Autodesk Inventor part; units mm, degrees
ref_plane "YZ Plane" through (0, 0, 0) normal (1, 0, 0) x (0, 1, 0)
ref_plane "XZ Plane" through (0, 0, 0) normal (0, 1, 0) x (-1, 0, 0)
ref_plane "XY Plane" through (0, 0, 0) normal (0, 0, 1) x (1, 0, 0)
ref_plane "Work Plane1" through (0, 0, 0) normal (0, 0, 1) x (1, 0, 0)
sketch "Sketch1" plane through (0, 0, 0) normal (0, 0, 1) x (1, 0, 0)
  circle A0 centre (0, -11.4) radius 0.5 construction
  circle A1 centre (0, 8.1) radius 0.5 construction
  circle A2 centre (0, -1.6) radius 3.9462 construction
  line L0 (8.2, 14.1) -> (-8.2, 14.1) construction
  line L1 (-8.2, 14.1) -> (-8.2, -14.1) construction
  line L2 (-8.2, -14.1) -> (8.2, -14.1) construction
  line L3 (8.2, -14.1) -> (8.2, 14.1) construction
  line L4 (-4, -9.1) -> (4, -9.1)
  line L5 (4, -9.1) -> (4, 5.9)
  line L6 (4, 5.9) -> (-4, 5.9)
  line L7 (-4, 5.9) -> (-4, -9.1)
  line L8 (-4, -9.1) -> (4, 5.9) construction
  line L9 (4, -9.1) -> (-4, 5.9) construction
  circle A3 centre (13, 11.4) radius 1.45 construction
  circle A4 centre (13, -14.6) radius 1.45 construction
  circle A5 centre (-20, -1.6) radius 1.45 construction
  line L10 (16, -17.6) -> (16, 14.4) construction
  line L11 (16, 14.4) -> (-16, 14.4) construction
  line L12 (-16, -17.6) -> (16, -17.6) construction
  line L13 (16, 14.4) -> (-24, 14.4)
  line L14 (-24, 14.4) -> (-24, -17.6)
  line L15 (-24, -17.6) -> (16, -17.6)
  line L16 (16, -17.6) -> (16, 14.4)
  circle A6 centre (0, 8.1) radius 0.5
  circle A7 centre (0, -11.4) radius 0.5
  point P0 (0, 0)
extrude "Extrusion1" add sketch "Sketch1" along normal blind 5
ref_plane "Work Plane2" through (-24, -1.6, 0) normal (0, -1, 0) x (1, 0, 0)
sketch "Sketch2" plane through (-24, -1.6, 0) normal (0, -1, 0) x (1, 0, 0)
  line L0 (1, 9) -> (1, 5)
  line L1 (7, 9) -> (7, 5)
  circle A0 centre (4, 4) radius 2.55
  line L2 (4, 6.55) -> (4, 1.45)
  point P0 (24, 0)
  dimension "d6" = 5.1
  dimension "d7" = 3
  dimension "d8" = 1
revolve "Revolution1" cut sketch "Sketch2" angle 360 about axis through (-20, -1.6, 6.55) along (0, 0, -1) picked at (3.097, 3.5418) contours L2 A0
sketch "Sketch3" plane through (0, 0, 5) normal (0, 0, 1) x (1, 0, 0)
  circle A0 centre (13, -14.6) radius 1.45
  circle A1 centre (13, 11.4) radius 1.45
  circle A2 centre (-20, -1.6) radius 1.45
  point P0 (0, 0)
ref_plane "Work Plane3" through (13, 11.4, 5) normal (0, 1, 0) x (1, 0, 0)
sketch "Sketch4" plane through (13, 11.4, 5) normal (0, 1, 0) x (1, 0, 0)
  circle A0 centre (0, 1) radius 2.55
  line L0 (-37, 0) -> (3, 0)
  line L1 (0, -4) -> (0, 0)
  line L2 (0, 0) -> (0, 3.55)
  line L3 (0, -1.55) -> (0, 0)
  point P0 (-13, 5)
  dimension "d10" = 5.1
  dimension "d11" = 1
  dimension "d12" = 0
revolve "Revolution2" cut sketch "Sketch4" angle 360 about axis through (13, 11.4, 5) along (0, 0, -1) picked at (-0.2076, 2.3409) picked at (-1.4654, -0.1719) contours L2 L0 A0 | L0 L1 A0
ref_plane "Work Plane4" through (13, -14.6, 5) normal (0, -1, 0) x (1, 0, 0)
sketch "Sketch5" plane through (13, -14.6, 5) normal (0, -1, 0) x (1, 0, 0)
  line L0 (0, 4) -> (0, 0)
  arc A0 (0, -3.55) -> (0, 1.55) centre (0, -1) ccw
  line L1 (0, 1.55) -> (0, -3.55)
  arc A1 (-2.3457, 0) -> (2.3457, 0) centre (0, -1) ccw
  point P0 (-13, -5)
  dimension "d14" = 5.1
  dimension "d15" = 1
revolve "Revolution3" cut sketch "Sketch5" angle 360 about axis through (13, -14.6, 9) along (0, 0, -1)
properties part number "05_Adapterplate_LG_CRD_8521B"
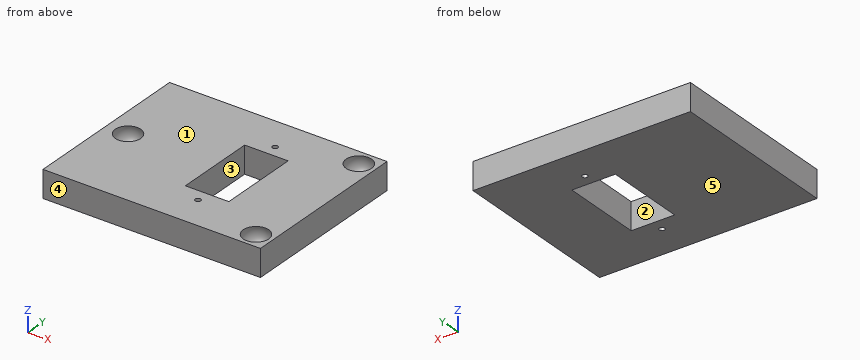
CAD build for the part. Positions are in the model's coordinates, mm. Face numbers are marked on the shaded views. A direction names the side the tool comes from. Round coordinates to 2 decimals unless told otherwise and drop trailing zeros. Write each loop counter-clockwise with the first axis right and the second up, starting at its lowest first coordinate (ties: lowest second). Pieces come first, ordered by that corner, then holes.
(1) Slice it at B-B, the plane x = 0. Write the cut outline in (y, z).
(2) Slice it at C-C, the plane z = 0.5. Write the cut outline in (x, y).
(3) 3-axis set-ups, long thin cutter, end or side, ignore diameter. For the marked faces 1 and 2: which of +Z, -Z, +X, -X, +Y, -Y reach the whole face in a straight line?
(4) Slice it at A-A, the plane y = 4.5. Write the cut outline in (x, z).
(5) Probe line 1 along Y through (x, z) = (0, 3.4); line 2 along X through (y, z) = (4, 3.15); line 3 along Y through (x, z) = (12, 1.95). List the from-to ranges inside material, lowest first.
(6) Mould opens along Y. For the marked faces 3, 4 and 5 say: pulls with the +Y half, pulls with the -Y half, needs draft (parallel to the pull), parting line crosses it, or undercut.
(7) Slice it at D-D, the plane z = 2.65. Write the cut outline in (x, y), and give its area (3 significant figures).
From the geometry:
1. outline: (-17.6, 0) - (-11.9, 0) - (-11.9, 5) - (-17.6, 5) - close; (-10.9, 0) - (-9.1, 0) - (-9.1, 5) - (-10.9, 5) - close; (5.9, 0) - (7.6, 0) - (7.6, 5) - (5.9, 5) - close; (8.6, 0) - (14.4, 0) - (14.4, 5) - (8.6, 5) - close
2. outline: (-24, -17.6) - (16, -17.6) - (16, 14.4) - (-24, 14.4) - close; hole (-4, -9.1) - (4, -9.1) - (4, 5.9) - (-4, 5.9) - close; hole circle Ø1 at (0, -11.4); hole circle Ø1 at (0, 8.1)
3. face 1: +Z, +X, -X, +Y, -Y
3. face 2: +Z, -Z
4. outline: (-24, 0) - (-4, 0) - (-4, 5) - (-24, 5) - close; (4, 0) - (16, 0) - (16, 5) - (4, 5) - close
5. line 1: y = -17.6 to -11.9, -10.9 to -9.1, 5.9 to 7.6, 8.6 to 14.4
5. line 2: x = -24 to -4, 4 to 16
5. line 3: y = -17.6 to -15.74, -13.46 to 10.26, 12.54 to 14.4
6. face 3: undercut
6. face 4: pulls with the -Y half
6. face 5: needs draft
7. outline: (-24, -17.6) - (16, -17.6) - (16, 14.4) - (-24, 14.4) - close; hole circle Ø4.33 at (-20, -1.6); hole (-4, -9.1) - (4, -9.1) - (4, 5.9) - (-4, 5.9) - close; hole circle Ø1 at (0, -11.4); hole circle Ø1 at (0, 8.1); hole circle Ø4.33 at (13, -14.6); hole circle Ø4.33 at (13, 11.4)
7. area: 1,110 mm2
